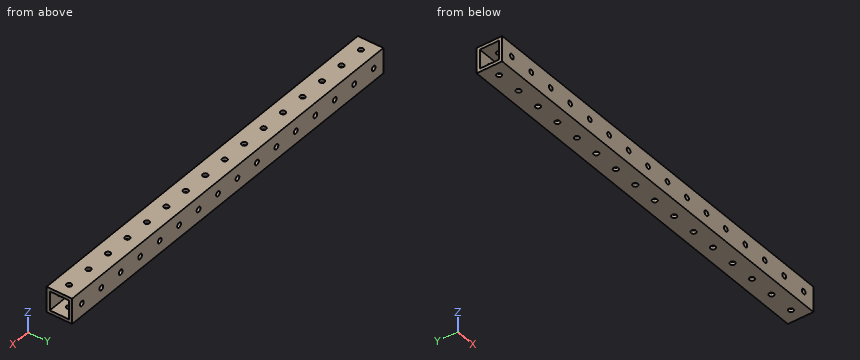
```python
from build123d import *

# Parameters (mm, degrees)
SKETCH1_W             = 25.4
SKETCH1_H             = 25.4
SKETCH1_W_2           = 19.05
SKETCH1_H_2           = 19.05
BOSS_EXTRUDE1_DEPTH   = 203.2
SKETCH3_W             = 2.4892
SKETCH3_H             = 25.4
SKETCH3_AT_POINT_2_W  = 2.4892
SKETCH3_AT_POINT_2_H  = 25.4
LPATTERN1_START       = -12.7
LPATTERN1_OUTLINE_R   = 2.4892
LPATTERN1_DEPTH       = 25.4
LPATTERN1_2_OUTLINE_R = 2.4892
LPATTERN1_2_DEPTH     = 25.4


# Read off the part's stored shape, not the designer's step: LPattern1
with BuildPart() as part:
    # Sketch1 → Boss-Extrude1 (new, symmetric)
    with BuildSketch(Plane(origin=(0, 0, 0), x_dir=(0, 0, -1), z_dir=(1, 0, 0))):
        Rectangle(SKETCH1_W, SKETCH1_H)
        Rectangle(SKETCH1_W_2, SKETCH1_H_2, mode=Mode.SUBTRACT)
    extrude(amount=BOSS_EXTRUDE1_DEPTH, both=True)

    # Sketch3 → #9 (0.196) Diameter Hole1 (revolve, cut)
    with BuildSketch(Plane(origin=(190.5, 12.7, 0), x_dir=(0, 0, 1), z_dir=(1, 0, 0))):
        with Locations((1.2446, 12.7)):
            Rectangle(SKETCH3_W, SKETCH3_H)
    revolve(axis=Axis((190.5, 19.05, 0), (0, -1, 0)), mode=Mode.SUBTRACT)

    # Sketch3 at point 2 (carried to point 2, square into its face) → #9 (0.196) Diameter Hole1 at 2 (revolve, cut)
    with BuildSketch(Plane(origin=(190.5, 0, 12.7), x_dir=(0, -1, 0), z_dir=(1, 0, 0))):
        with Locations((1.2446, 12.7)):
            Rectangle(SKETCH3_AT_POINT_2_W, SKETCH3_AT_POINT_2_H)
    revolve(axis=Axis((190.5, 0, 19.05), (0, 0, -1)), mode=Mode.SUBTRACT)

    # LPattern1 outline → LPattern1 (cut)
    with BuildSketch(Plane.XY.offset(LPATTERN1_START)):
        with Locations((165.1, 0)):
            Circle(LPATTERN1_OUTLINE_R)
        with Locations((139.7, 0)):
            Circle(LPATTERN1_OUTLINE_R)
        with Locations((114.3, 0)):
            Circle(LPATTERN1_OUTLINE_R)
        with Locations((88.9, 0)):
            Circle(LPATTERN1_OUTLINE_R)
        with Locations((63.5, 0)):
            Circle(LPATTERN1_OUTLINE_R)
        with Locations((38.1, 0)):
            Circle(LPATTERN1_OUTLINE_R)
        with Locations((12.7, 0)):
            Circle(LPATTERN1_OUTLINE_R)
        with Locations((-12.7, 0)):
            Circle(LPATTERN1_OUTLINE_R)
        with Locations((-38.1, 0)):
            Circle(LPATTERN1_OUTLINE_R)
        with Locations((-63.5, 0)):
            Circle(LPATTERN1_OUTLINE_R)
        with Locations((-88.9, 0)):
            Circle(LPATTERN1_OUTLINE_R)
        with Locations((-114.3, 0)):
            Circle(LPATTERN1_OUTLINE_R)
        with Locations((-139.7, 0)):
            Circle(LPATTERN1_OUTLINE_R)
        with Locations((-165.1, 0)):
            Circle(LPATTERN1_OUTLINE_R)
        with Locations((-190.5, 0)):
            Circle(LPATTERN1_OUTLINE_R)
    extrude(amount=LPATTERN1_DEPTH, mode=Mode.SUBTRACT)

    # LPattern1 2 outline → LPattern1 2 (cut)
    with BuildSketch(Plane(origin=(0, 0, 0), x_dir=(1, 0, 0), z_dir=(0, 1, 0)).offset(LPATTERN1_START)):
        with Locations((165.1, 0)):
            Circle(LPATTERN1_2_OUTLINE_R)
        with Locations((139.7, 0)):
            Circle(LPATTERN1_2_OUTLINE_R)
        with Locations((114.3, 0)):
            Circle(LPATTERN1_2_OUTLINE_R)
        with Locations((88.9, 0)):
            Circle(LPATTERN1_2_OUTLINE_R)
        with Locations((63.5, 0)):
            Circle(LPATTERN1_2_OUTLINE_R)
        with Locations((38.1, 0)):
            Circle(LPATTERN1_2_OUTLINE_R)
        with Locations((12.7, 0)):
            Circle(LPATTERN1_2_OUTLINE_R)
        with Locations((-12.7, 0)):
            Circle(LPATTERN1_2_OUTLINE_R)
        with Locations((-38.1, 0)):
            Circle(LPATTERN1_2_OUTLINE_R)
        with Locations((-63.5, 0)):
            Circle(LPATTERN1_2_OUTLINE_R)
        with Locations((-88.9, 0)):
            Circle(LPATTERN1_2_OUTLINE_R)
        with Locations((-114.3, 0)):
            Circle(LPATTERN1_2_OUTLINE_R)
        with Locations((-139.7, 0)):
            Circle(LPATTERN1_2_OUTLINE_R)
        with Locations((-165.1, 0)):
            Circle(LPATTERN1_2_OUTLINE_R)
        with Locations((-190.5, 0)):
            Circle(LPATTERN1_2_OUTLINE_R)
    extrude(amount=LPATTERN1_2_DEPTH, mode=Mode.SUBTRACT)


solid = part.part
```
Here's how the part is built. I have some questions about the finished solid (model axes, mm). Give positions to 0.01 mm unless a question says otherwise; leave off trailing zeros. Order: outer loops, then holes, each group sorted by start corner. A loop starts at its lowest first (then second) coordinate and runs counter-clockwise, first axis right, second up. Notation, with made-up numbers: M 89.5,17.5 L 111.5,17.5 A19 ccw 111.5,38.5 Z; hole C 85,29 d6. An arc over 180 degrees is marked long. Use a Markdown table: item, result. Add a question column.
1. Suppose I cut it at A-A (x = -23.5). List the corners of the cut face in (y, z) for me (3 decimals).
2. For pin 1 Ø4.5 at (x, y) = (-38.1, 0) entering from -Z, with a flat end and sliding along its axis, tell me the tip position at first contact or that it passes through.
3. I need wall thicknesses on probe 1 along Y at (x, z) = (92.5, -0.5) (3 decimals); probe 2 along Z at (x, y) = (-139.7, 11.35). Which ranges of each line are inside material? Lowest first, please. Write a range as from..to.
Results list:
| question | item | result |
|---|---|---|
| 1 | outline | M -12.7,-12.7 L 12.7,-12.7 L 12.7,12.7 L -12.7,12.7 Z; hole M -9.525,-9.525 L 9.525,-9.525 L 9.525,9.525 L -9.525,9.525 Z |
| 2 | pin 1 | passes through |
| 3 | probe 1 | y = -12.7..-9.525, 9.525..12.7 |
| 3 | probe 2 | z = -12.7..-2.49, 2.49..12.7 |
